Verification items for the finished model (mm, model axes). A direction names the side the tool comes from. Coordinates: 2 decimals unless noted, no trailing zeros. Use CSV: the item, a comma, the result in double quotes. Start each with the question number.
```python
from build123d import *

# Parameters (mm, degrees)
F1_DEPTH = 10
F2_W     = 10.5
F2_H     = 8.5
F3_DEPTH = 10
F4_R     = 1.125
F5_DEPTH = 5.7948195458


with BuildPart() as f1:
    # F0 (on Top) → F1 (new body)
    with BuildSketch(Plane.XY):
        with BuildLine():
            add(Edge.make_bspline(
                [(-70, -120), (-69.9490740645, -72.2301395677), (0.3708027655, 112.2301395677), (69.2074685334, -72.2301395677), (70, -120)],
                knots=[0, 0, 0, 0, 0.5, 1, 1, 1, 1], degree=3))
            Line((-70, -120), (-60, -120))
            add(Edge.make_bspline(
                [(-60, -120), (-60.2770864151, -94.6751633451), (0.1071934019, 94.6751633451), (60.0626996113, -94.6751633451), (60, -120)],
                knots=[0, 0, 0, 0, 0.5, 1, 1, 1, 1], degree=3))
            Line((60, -120), (70, -120))
        make_face()
    extrude(amount=F1_DEPTH)

    # F2 (on face) → F3 (cut, through all)
    with BuildSketch(Plane.XY.offset(10)):
        with Locations((0, 10)):
            Rectangle(F2_W, F2_H)
    extrude(amount=-F3_DEPTH, mode=Mode.SUBTRACT)

    # F4 (on face) → F5 (cut, through all)
    with BuildSketch(Plane(origin=(0, 5.75, 0), x_dir=(-1, 0, 0), z_dir=(0, 1, 0))):
        with Locations((0, 5)):
            Circle(F4_R)
    extrude(amount=-F5_DEPTH, mode=Mode.SUBTRACT)


solid = f1.part
```
Q1. Tool access check on faces 3 (the flat face through (65, -120, 5)), 4 (the flat face through (-1, 5.75, 6)). Record the directions out of +Z, -Z, +X, -X, +Y, -Y that give a thin tool (end or side, any length) a straight path to the whole face; none if there is none.
Q2. Release check for a two-part mould opening along X. For faces 1 (the flat face through (0, 14.25, 5)), 2 (the flat face through (26.3, -20.5, 10)) record: released by +X, released by -X, zero draft, split by the parting line, or undercut.
Q3. Scan lines: line 1 along Z through (x, y) = (0, 2) (3 decimals); line 2 along X through (y, z) = (2.35, 5) (3 decimals); line 3 along X through (y, z) = (2.8, 5) (3 decimals). Record each from-to range of solid material in increasing order. Write a range as from..to.
Q4. Gauge pin test, flat ends, axial feed: pin 1 (1.5 mm diameter, centred on x = -32, z = 8.5, fed in from -Y); pin 2 (1.3 mm diameter, centred on x = 0, z = 5, fed in from -Y); pin 3 (2 mm diameter, centred on x = -55, y = -103, fed in from +Z); pin 4 (3 mm diameter, centred on x = 1, z = 6.5, fed in from -Y). Record the tip position at first contact, or that the pin passes through.
Reply:
1,face 3,"+Z, -Z, +X, -X, -Y"
1,face 4,"+Z, -Z"
2,face 1,"undercut"
2,face 2,"zero draft"
3,line 1,"0..3.875, 6.125..10"
3,line 2,"-27.7..-1.125, 1.125..27.58"
3,line 3,"-27.333..-1.125, 1.125..27.216"
4,pin 1,"y = -32.17"
4,pin 2,"y = 14.25"
4,pin 3,"through"
4,pin 4,"y = -0.21"
